from build123d import *

# Parameters (mm, degrees)
SKETCH1_W           = 48
SKETCH1_H           = 19
BOSS_EXTRUDE1_DEPTH = 2
SKETCH2_R           = 2
SKETCH2_R_2         = 1
BOSS_EXTRUDE2_DEPTH = 6
CUT_EXTRUDE1_REACH  = 53.971
SKETCH3_R           = 1.5


with BuildPart() as part:
    # Sketch1 → Boss-Extrude1 (new body)
    with BuildSketch(Plane.YZ):
        with Locations((24, 9.5)):
            Rectangle(SKETCH1_W, SKETCH1_H)
    extrude(amount=BOSS_EXTRUDE1_DEPTH)

    # Sketch2 → Boss-Extrude2 (add)
    # profile 1 of 2: a face of its own
    with BuildSketch(Plane(origin=(0, 0, 0), x_dir=(0, -1, 0), z_dir=(-1, 0, 0))):
        with Locations(Location((-46, 17, 0), (0, 0, 90))):
            Circle(SKETCH2_R)
        with Locations(Location((-46, 17, 0), (0, 0, 90))):
            Circle(SKETCH2_R_2, mode=Mode.SUBTRACT)
    # profile 2 of 2: a face of its own
    with BuildSketch(Plane(origin=(0, 0, 0), x_dir=(0, -1, 0), z_dir=(-1, 0, 0))):
        with Locations(Location((-2, 2, 0), (0, 0, 270))):
            Circle(SKETCH2_R)
        with Locations(Location((-2, 2, 0), (0, 0, 90))):
            Circle(SKETCH2_R_2, mode=Mode.SUBTRACT)
    extrude(amount=BOSS_EXTRUDE2_DEPTH)

    # Sketch3 → Cut-Extrude1 (cut, up to next)
    with BuildSketch(Plane(origin=(0, 0, 0), x_dir=(0, -1, 0), z_dir=(-1, 0, 0)), mode=Mode.PRIVATE) as cut_extrude1_sk1:
        with Locations(Location((-42, 6, 0), (0, 0, 90))):
            Circle(SKETCH3_R)
    cut_extrude1_tool1 = extrude(cut_extrude1_sk1.sketch, amount=-CUT_EXTRUDE1_REACH, mode=Mode.PRIVATE) & part.part
    add(cut_extrude1_tool1.solids().sort_by_distance((0, 42, 6))[0], mode=Mode.SUBTRACT)


solid = part.part
Build history of the part. All positions in model axes, mm. A direction names the side the tool comes from. Round coordinates to 2 decimals unless told otherwise and drop trailing zeros. Order: outer loops, then holes, each group sorted by start corner. A loop starts at its lowest first (then second) coordinate and runs counter-clockwise, first axis right, second up. Notation, with made-up numbers: M 20,15.5 L 70,15.5 A28 ccw 70,42.5 Z; hole C 55,0.5 d4. An arc over 180 degrees is marked long. Use CSV: the item, a comma, the result in double quotes. Start each with the question number.
(1) Cut at D-D on y = 12. List the corners of the cut face in (x, z), then the cut area to 3 significant figures.
(2) Flat gauge pin, fed straight in: P1, Ø1, axis at y = 46, z = 17, coming from the -X side. Where does the tip first touch, or does it go through?
(3) Mould opens along Z. For faces 1 (the face through (0, 0.4, 0.5)), 2 (the face through (1, 24, 19)), 3 (the face through (0, 46, 17)) say: +Z half, -Z half, draft (parallel to the pull), parting line (faces both ways), or undercut.
(4) Cut at C-C on x = -5. List the corners of the cut face in (y, z), then the cut area to 3 significant figures.
(5) Tool access for faces 4 (the face through (0, 47.5, 18.6)), 5 (the face through (0, 2, 2)), 6 (the face through (-6, 45, 18)): list every direction of +Z, -Z, +X, -X, +Y, -Y with a clear straight run to the whole face (end or side of a thin tool).
(6) Cut at A-A on y = 42. List the corners of the cut face in (x, z), then the cut area to 3 significant figures.
(7) Drill centre lines: probe 1 along Y at (x, z) = (-1.95, 2); probe 2 along Y at (x, z) = (-3.55, 17); probe 3 along X at (y, z) = (46, 8.75). Where is each one in solid material? Low to high.
(8) Cut at B-B on z = 6. List the corners of the cut face in (x, y), then the cut area to 3 significant figures.
Findings:
1,outline,"M 0,0 L 2,0 L 2,19 L 0,19 Z"
1,area,"38.0 mm^2"
2,P1,"stops at x = 0"
3,face 1,"draft"
3,face 2,"+Z half"
3,face 3,"undercut"
4,outline,"C 2,2 d4; C 46,17 d4; hole C 2,2 d2; hole C 46,17 d2"
4,area,"18.8 mm^2"
5,face 4,"+Z, -X, +Y"
5,face 5,"-X"
5,face 6,"+Z, -Z, -X, +Y, -Y"
6,outline,"M 0,0 L 2,0 L 2,4.5 L 0,4.5 Z; M 0,7.5 L 2,7.5 L 2,19 L 0,19 Z"
6,area,"32.0 mm^2"
7,probe 1,"y = 0 to 1, 3 to 4"
7,probe 2,"y = 44 to 45, 47 to 48"
7,probe 3,"x = 0 to 2"
8,outline,"M 0,0 L 2,0 L 2,40.5 L 0,40.5 Z; M 0,43.5 L 2,43.5 L 2,48 L 0,48 Z"
8,area,"90.0 mm^2"
